CAD build for the part. Positions are in the model's coordinates, mm. A direction names the side the tool comes from. Coordinates: 2 decimals unless noted, no trailing zeros. Write each loop counter-clockwise with the first axis right and the second up, starting at its lowest first coordinate (ties: lowest second). Pieces come first, ordered by that corner, then holes. Notation, with made-up numbers: (-14.5, 26) -> (6.5, 26) arc R32 cw to (6.5, 61) -> close; hole circle Ø3 at (-20.5, 9). An arc over 180 degrees is marked (long way). Answer as CSV lines item,"result".
```python
from build123d import *

# Parameters (mm, degrees)
BOSS_EXTRUDE1_DEPTH = 10
SKETCH3_R           = 4
BOSS_EXTRUDE2_DEPTH = 43
SKETCH4_R           = 2.5
CUT_EXTRUDE1_DEPTH  = 5
SKETCH6_R           = 12.5
BOSS_EXTRUDE3_DEPTH = 5
CUT_EXTRUDE2_START  = -5
SKETCH7_R           = 2.5
CUT_EXTRUDE2_DEPTH  = 5


with BuildPart() as part:
    # Sketch1 → Boss-Extrude1 (new, symmetric)
    with BuildSketch(Plane.XY):
        with BuildLine():
            Line((-22.5, 0), (-14.95, 60))
            Line((-14.95, 60), (14.95, 60))
            Line((14.95, 60), (22.5, 0))
            ThreePointArc((22.5, 0), (0, -22.5), (-22.5, 0))
        make_face()
    extrude(amount=BOSS_EXTRUDE1_DEPTH, both=True)

    # Sketch3 → Boss-Extrude2 (add)
    with BuildSketch(Plane(origin=(0, 60, 0), x_dir=(1, 0, 0), z_dir=(0, 1, 0))):
        with Locations(Location((0, 0, 0), (0, 0, 270))):
            Circle(SKETCH3_R)
    extrude(amount=BOSS_EXTRUDE2_DEPTH)

    # Sketch4 → Cut-Extrude1 (cut)
    with BuildSketch(Plane.XY.offset(10)):
        Circle(SKETCH4_R)
    extrude(amount=-CUT_EXTRUDE1_DEPTH, mode=Mode.SUBTRACT)

    # Sketch6 → Boss-Extrude3 (add)
    with BuildSketch(Plane(origin=(0, 0, -10), x_dir=(-1, 0, 0), z_dir=(0, 0, -1))):
        with Locations(Location((0, 0, 0), (0, 0, 180))):
            Circle(SKETCH6_R)
    extrude(amount=BOSS_EXTRUDE3_DEPTH)

    # Sketch7 → Cut-Extrude2 (cut)
    with BuildSketch(Plane(origin=(0, 0, -15), x_dir=(-1, 0, 0), z_dir=(0, 0, -1)).offset(CUT_EXTRUDE2_START)):
        with Locations(Location((0, 0, 0), (0, 0, 180))):
            Circle(SKETCH7_R)
    extrude(amount=CUT_EXTRUDE2_DEPTH, mode=Mode.SUBTRACT)


solid = part.part
```
Item 1: Flat gauge pins, fed straight in: pin 1 (8 mm diameter, centred on x = 4.5, z = 3.5, fed in from -Y); pin 2 (5.5 mm diameter, centred on x = 0.5, y = -1, fed in from +Z); pin 3 (12 mm diameter, centred on y = 51, z = 0, fed in from -X); pin 4 (3 mm diameter, centred on x = 0, y = 0, fed in from -Z). Where does each tip first touch, or does it go through?
Answer below:
pin 1,"stops at y = -22.49"
pin 2,"stops at z = 10"
pin 3,"stops at x = -16.84"
pin 4,"stops at z = -10"
Item 2: 3-axis set-ups, long thin cutter, end or side, ignore diameter. For faces 5 (the cylindrical face through (-0.54, -2.44, 7.54)), 6 (the flat face through (-4, 60, -2)), 7 (the cylindrical face through (11.923, -3.755, -12.465)): which of +Z, -Z, +X, -X, +Y, -Y reach the whole face in a straight line?
Answer below:
face 5,"+Z"
face 6,"+Y"
face 7,"-Z"
Item 3: Saw through at C-C on y = 7. Give the cut face in (x, z).
Answer below:
outline,"(-21.62, -10) -> (-10.36, -10) -> (-10.36, -15) -> (10.36, -15) -> (10.36, -10) -> (21.62, -10) -> (21.62, 10) -> (-21.62, 10) -> close"
Item 4: Two-plate mould, pull along Y, no slides. Class faces 1 (the cylindrical face through (0.495, -22.495, 0.14)), 2 (the cylindrical face through (-3.905, 81.199, -0.867)), 3 (the cylindrical face through (-2.5, -0.1, -12.5)), 4 (the flat face through (0, 0, -10)): pulls with the +Y half, pulls with the -Y half, needs draft (parallel to the pull), parting line crosses it, or undercut.
Answer below:
face 1,"pulls with the -Y half"
face 2,"needs draft"
face 3,"undercut"
face 4,"undercut"
Item 5: Saw through at B-B on z = 0. Give the cut face in (x, y), and give its area (3 significant figures).
Answer below:
outline,"(-22.5, 0) arc R22.5 ccw to (22.5, 0) -> (14.95, 60) -> (4, 60) -> (4, 103) -> (-4, 103) -> (-4, 60) -> (-14.95, 60) -> close"
area,"3,390 mm2"
Item 6: Wall check: line 1 (Y direction, x = 0, z = 8.45); line 2 (Y direction, x = 0, z = -13.9); line 3 (Z direction, x = -3, y = 45). Give the ranges that are in metal, low to high. Write a range as from..to.
Answer below:
line 1,"y = -22.5..-2.5, 2.5..60"
line 2,"y = -12.5..-2.5, 2.5..12.5"
line 3,"z = -10..10"
Item 7: Saw through at A-A on x = 0. Give the cut face in (y, z).
Answer below:
outline,"(-22.5, -10) -> (-12.5, -10) -> (-12.5, -15) -> (-2.5, -15) -> (-2.5, -10) -> (2.5, -10) -> (2.5, -15) -> (12.5, -15) -> (12.5, -10) -> (60, -10) -> (60, -4) -> (103, -4) -> (103, 4) -> (60, 4) -> (60, 10) -> (2.5, 10) -> (2.5, 5) -> (-2.5, 5) -> (-2.5, 10) -> (-22.5, 10) -> close"
Item 8: Saw through at D-D on z = -8.5. Give the cut face in (x, y), and give its area (3 significant figures).
Answer below:
outline,"(-22.5, 0) arc R22.5 ccw to (22.5, 0) -> (14.95, 60) -> (-14.95, 60) -> close"
area,"3,040 mm2"
